The figure shows three views and two pictorial views of one solid part (mm, origin at its lowest corner). Answer the questions. Coordinates: 2 decimals unless noted, no trailing zeros. Loops run counter-clockwise (first coordinate to the right, second up) from the corner with the lowest first, then second, coordinate; pieces in that order, holes last. Notation, with made-up numbers: M 67.25,16.25 L 119.25,16.25 A23 cw 119.25,47.25 Z; hole C 5.25,43 d6. An arc over 180 degrees is marked long. Answer as a JSON object with one key per item and string values. Group by question number.
1. A cutting plane is placed at D-D on y = 621. Give the vertices of the cut face in (x, z), and give its area (3 significant figures).
2. A cutting plane is placed at A-A on z = 436. Give the vertices of the cut face in (x, y), and give its area (3 significant figures).
3. Determine the mould class of the marked faces 1 and 2 for opening direction Y: released by +Y, released by -Y, zero draft, split by the parting line, or undercut.
4. A cutting plane is placed at C-C on x = 708. Give the vertices of the cut face in (y, z), and give its area (3 significant figures).
5. A cutting plane is placed at B-B on y = 1024.5. Give the vertices of the cut face in (x, z), and give its area (3 significant figures).
6. Straight lines are drawn through the part: L1, parallel to X at y = 213.5, z = 188; L2, parallel to Z at x = 369.5, y = 850. For each, find the intervals that lie inside material, in ascending order.
7. Given pin 1 (24 mm diameter, centred on x = 214.5, z = 451, fed in from +Y); pin 2 (3 mm diameter, centred on x = 736.5, y = 825, fed in from -Z); pin 3 (1 mm diameter, centred on y = 1011.5, z = 316.5, fed in from -X); pin 4 (24 mm diameter, centred on x = 194, z = 403, fed in from -Y), each flat-ended and moving along its own axis, determine where each tip first touches the part or whether it passes through.
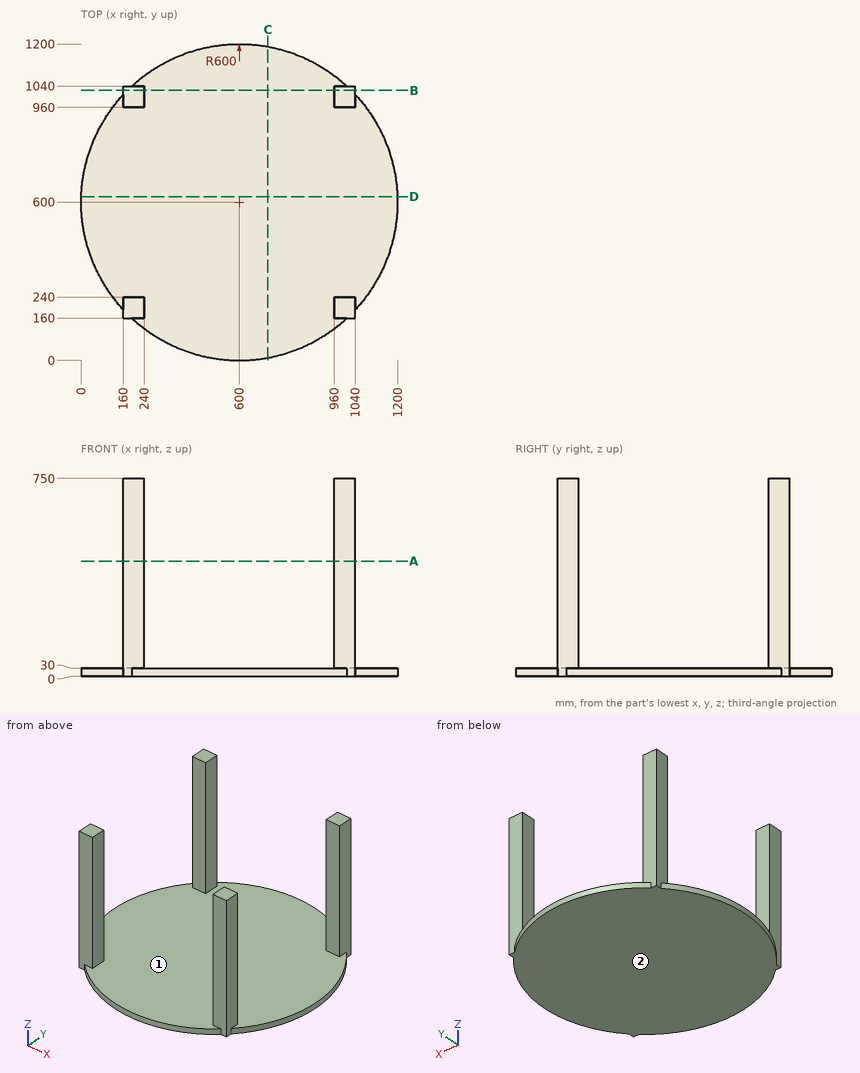
From the geometry:
{
 "1": {"outline": "M 0.37,0 L 1199.63,0 L 1199.63,30 L 0.37,30 Z", "area": "36,000 mm²"},
 "2": {"outline": "M 160,160 L 240,160 L 240,240 L 160,240 Z; M 160,960 L 240,960 L 240,1040 L 160,1040 Z; M 960,160 L 1040,160 L 1040,240 L 960,240 Z; M 960,960 L 1040,960 L 1040,1040 L 960,1040 Z", "area": "25,600 mm²"},
 "3": {"face 1": "undercut", "face 2": "zero draft"},
 "4": {"outline": "M 9.8,0 L 1190.2,0 L 1190.2,30 L 9.8,30 Z", "area": "35,400 mm²"},
 "5": {"outline": "M 160,0 L 1040,0 L 1040,750 L 960,750 L 960,30 L 240,30 L 240,750 L 160,750 Z", "area": "142,000 mm²"},
 "6": {"L1": "x = 160 to 240, 960 to 1040", "L2": "z = 0 to 30"},
 "7": {"pin 1": "stops at y = 1040", "pin 2": "stops at z = 0", "pin 3": "stops at x = 160", "pin 4": "stops at y = 160"}
}
